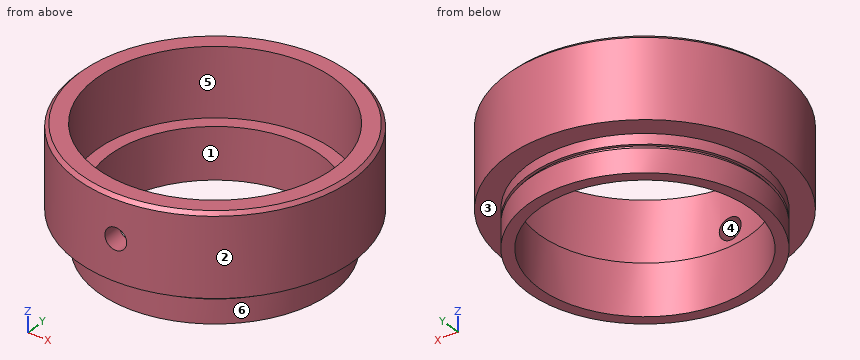
```python
from build123d import *

# Parameters (mm, degrees)
SKETCH2_R          = 1.6
CUT_EXTRUDE1_DEPTH = 25


with BuildPart() as part:
    # Sketch1 → Revolve1 (revolve)
    with BuildSketch(Plane(origin=(0, 0, 0), x_dir=(1, 0, 0), z_dir=(0, 1, 0))):
        Polygon((-17.45, 0), (-19.8, 0), (-20.3, 0.5), (-20.3, 12), (-17.160824742, 12), (-17.160824742, 13.5), (-16.760824742, 13.5), (-16.760824742, 14), (-17.160824742, 14), (-17.160824742, 17.5), (-15.50386168, 17.5), (-15.50386168, 10), (-17.45, 10), align=None)
    revolve(axis=Axis((0, 0, 0), (0, 0, -1)))

    # Sketch2 → Cut-Extrude1 (cut)
    with BuildSketch(Plane(origin=(0, 0, 0), x_dir=(1, 0, 0), z_dir=(0, 1, 0))):
        with Locations((0, 6)):
            Circle(SKETCH2_R)
    extrude(amount=-CUT_EXTRUDE1_DEPTH, mode=Mode.SUBTRACT)


solid = part.part
```
Work out the finished part from the listing and answer in its coordinate system (mm). Face numbers are marked on the shaded views. A direction names the side the tool comes from. Round coordinates to 2 decimals unless told otherwise and drop trailing zeros. Write each loop counter-clockwise with the first axis right and the second up, starting at its lowest first coordinate (ties: lowest second). Pieces come first, ordered by that corner, then holes.
1) A cutting plane is placed at B-B on x = 0. Give the number of separate pieces and of enclosed holes in the cut face, and give its area (3 significant figures).
2) A cutting plane is placed at D-D on z = -6.75. Determine the outline of the cut face in (x, y), and give its area (3 significant figures).
3) A cutting plane is placed at A-A on y = 0. Determine the outline of the cut face in (x, z).
4) A cutting plane is placed at C-C on z = -1.75. Determine the outline of the cut face in (x, y).
5) Determine the mould class of the marked faces 1, 2 and 3 for opening direction X: pulls with the +X half, pulls with the -X half, needs draft (parallel to the pull), parting line crosses it, or undercut.
6) Consider probe 1 along Y at (x, z) = (0, -12.25); probe 2 along Y at (x, z) = (0, -3); probe 3 along Z at (x, y) = (-13, -10). Determine where each line is inside the solid, lowest interval first.
7) Flat-ended cylindrical pins translate along their axes: P1, Ø10, axis at x = 6, z = -12, coming from the -Y side; P2, Ø8, axis at y = -10, z = -3.5, coming from the -X side; P3, Ø1.5, axis at y = -1, z = -9, coming from the -X side. Find the tip coordinate at first contact, or state that the pin passes through.
8) Which of the six approach directions +Z, -Z, +X, -X, +Y, -Y give full straight-line access (tool end or side, diameter ignored) to the marked faces 4, 5 and 6?
Entries:
1. separate pieces: 3
1. enclosed holes: 0
1. area: 84.6 mm2
2. outline: (-1.41, -20.25) - (-1.41, -17.39) arc R17.45 cw (long way) to (1.41, -17.39) - (1.41, -20.25) arc R20.3 ccw (long way) to start
2. area: 330 mm2
3. outline: (-20.3, -12) - (-17.16, -12) - (-17.16, -13.5) - (-16.76, -13.5) - (-16.76, -14) - (-17.16, -14) - (-17.16, -17.5) - (-15.5, -17.5) - (-15.5, -10) - (-17.45, -10) - (-17.45, 0) - (-19.8, 0) - (-20.3, -0.5) - close; (15.5, -17.5) - (17.16, -17.5) - (17.16, -14) - (16.76, -14) - (16.76, -13.5) - (17.16, -13.5) - (17.16, -12) - (20.3, -12) - (20.3, -0.5) - (19.8, 0) - (17.45, 0) - (17.45, -10) - (15.5, -10) - close
4. outline: circle Ø40.6 at (0, 0); hole circle Ø34.9 at (0, 0)
5. face 1: undercut
5. face 2: parting line crosses it
5. face 3: needs draft
6. probe 1: y = -17.16 to -15.5, 15.5 to 17.16
6. probe 2: y = -20.3 to -17.45, 17.45 to 20.3
6. probe 3: z = -17.5 to -10
7. P1: stops at y = -20.28
7. P2: stops at x = -19.39
7. P3: stops at x = -20.3
8. face 4: -Y
8. face 5: +Z
8. face 6: -Z
